```python
from build123d import *

# Parameters (mm, degrees)
SKETCH_1_W               = 120
SKETCH_1_H               = 15
EXTRUDE_1_DEPTH          = 8
FILLET_1_R               = 5
SKETCH_6_R               = 12.5
EXTRUDE_2_DEPTH          = 8
SKETCH_7_R               = 1
CUT_EXTRUDE_4_DEPTH      = 23
SKETCH_8_R               = 2.4
CUT_EXTRUDE_5_DEPTH      = 23
SKETCH_9_W               = 8
SKETCH_9_H               = 15
EXTRUDE_3_DEPTH          = 100
SKETCH_10_W              = 25
SKETCH_10_H              = 6
CUT_EXTRUDE_6_DEPTH      = 5
CUT_EXTRUDE_7_DEPTH      = 7
CUT_EXTRUDE_7_DEPTH_BACK = 15
SKETCH_4_R               = 1
FILLET_2_R               = 10
FILLET_4_R               = 5
CUT_EXTRUDE_8_REACH      = 123.918
SKETCH_12_R              = 1


with BuildPart() as part:
    # 草图1 → 凸台-拉伸1 (new body)
    with BuildSketch(Plane(origin=(0, 0, 0), x_dir=(0, 0, -1), z_dir=(1, 0, 0))):
        with Locations((60, 7.5)):
            Rectangle(SKETCH_1_W, SKETCH_1_H)
    extrude(amount=EXTRUDE_1_DEPTH)

    # 圆角1
    fillet_1_edges = [part.edges().sort_by_distance(p)[0] for p in [
        (4, 15, 0),
        (4, 15, -120),
        (4, 0, -120),
        (4, 0, 0),
    ]]
    fillet(fillet_1_edges, radius=FILLET_1_R)

    # 草图6 → 凸台-拉伸2 (add)
    with BuildSketch(Plane(origin=(8, 0, 0), x_dir=(0, 0, -1), z_dir=(1, 0, 0))):
        with Locations((6.4, 7.5)):
            Circle(SKETCH_6_R)
    extrude(amount=-EXTRUDE_2_DEPTH)

    # 草图7 → 切除-拉伸4 (cut)
    with BuildSketch(Plane.ZY):
        with Locations((-6.4, 12.5)):
            Circle(SKETCH_7_R)
        with Locations((-6.4, 2.5)):
            Circle(SKETCH_7_R)
    extrude(amount=-CUT_EXTRUDE_4_DEPTH, mode=Mode.SUBTRACT)

    # 草图8 → 切除-拉伸5 (cut)
    with BuildSketch(Plane.ZY):
        with Locations((-6.4, 7.5)):
            Circle(SKETCH_8_R)
    extrude(amount=-CUT_EXTRUDE_5_DEPTH, mode=Mode.SUBTRACT)

    # 草图9 → 凸台-拉伸3 (add)
    with BuildSketch(Plane.XY):
        with Locations((4, 7.5)):
            Rectangle(SKETCH_9_W, SKETCH_9_H)
    extrude(amount=EXTRUDE_3_DEPTH)

    # 草图10 → 切除-拉伸6 (cut)
    with BuildSketch(Plane.ZY):
        with Locations((16.022995474, 7.5)):
            Rectangle(SKETCH_10_W, SKETCH_10_H)
    extrude(amount=-CUT_EXTRUDE_6_DEPTH, mode=Mode.SUBTRACT)

    # 草图4 → 切除-拉伸7 (cut, two sides: drawn at the far end of the back side and taken through both)
    with BuildSketch(Plane.XY.offset(-CUT_EXTRUDE_7_DEPTH_BACK)):
        with Locations(Location((2.5, 7.5, 0), (0, 0, 180.000000002))):
            Circle(SKETCH_4_R)
    extrude(amount=CUT_EXTRUDE_7_DEPTH + CUT_EXTRUDE_7_DEPTH_BACK, mode=Mode.SUBTRACT)

    # 圆角2
    fillet_2_edges = [part.edges().sort_by_distance(p)[0] for p in [
        (4, 0, -16.4),
        (4, 15, -16.4),
        (4, 15, 3.6),
        (4, 0, 3.6),
    ]]
    fillet(fillet_2_edges, radius=FILLET_2_R)

    # 圆角4
    fillet_4_edges = [part.edges().sort_by_distance(p)[0] for p in [
        (4, 0, 100),
        (4, 15, 100),
    ]]
    fillet(fillet_4_edges, radius=FILLET_4_R)

    # 草图12 → 切除-拉伸8 (cut, up to next)
    with BuildSketch(Plane.ZY, mode=Mode.PRIVATE) as cut_extrude_8_sk1:
        with Locations((-115, 7.5)):
            Circle(SKETCH_12_R)
    cut_extrude_8_tool1 = extrude(cut_extrude_8_sk1.sketch, amount=-CUT_EXTRUDE_8_REACH, mode=Mode.PRIVATE) & part.part
    # 草图12 → 切除-拉伸8 (cut, up to next)
    with BuildSketch(Plane.ZY, mode=Mode.PRIVATE) as cut_extrude_8_sk2:
        with Locations((-105, 7.5)):
            Circle(SKETCH_12_R)
    cut_extrude_8_tool2 = extrude(cut_extrude_8_sk2.sketch, amount=-CUT_EXTRUDE_8_REACH, mode=Mode.PRIVATE) & part.part
    # 草图12 → 切除-拉伸8 (cut, up to next)
    with BuildSketch(Plane.ZY, mode=Mode.PRIVATE) as cut_extrude_8_sk3:
        with Locations((-82, 7.5)):
            Circle(SKETCH_12_R)
    cut_extrude_8_tool3 = extrude(cut_extrude_8_sk3.sketch, amount=-CUT_EXTRUDE_8_REACH, mode=Mode.PRIVATE) & part.part
    # 草图12 → 切除-拉伸8 (cut, up to next)
    with BuildSketch(Plane.ZY, mode=Mode.PRIVATE) as cut_extrude_8_sk4:
        with Locations((-72, 7.5)):
            Circle(SKETCH_12_R)
    cut_extrude_8_tool4 = extrude(cut_extrude_8_sk4.sketch, amount=-CUT_EXTRUDE_8_REACH, mode=Mode.PRIVATE) & part.part
    # 草图12 → 切除-拉伸8 (cut, up to next)
    with BuildSketch(Plane.ZY, mode=Mode.PRIVATE) as cut_extrude_8_sk5:
        with Locations((95, 7.5)):
            Circle(SKETCH_12_R)
    cut_extrude_8_tool5 = extrude(cut_extrude_8_sk5.sketch, amount=-CUT_EXTRUDE_8_REACH, mode=Mode.PRIVATE) & part.part
    # 草图12 → 切除-拉伸8 (cut, up to next)
    with BuildSketch(Plane.ZY, mode=Mode.PRIVATE) as cut_extrude_8_sk6:
        with Locations((85, 7.5)):
            Circle(SKETCH_12_R)
    cut_extrude_8_tool6 = extrude(cut_extrude_8_sk6.sketch, amount=-CUT_EXTRUDE_8_REACH, mode=Mode.PRIVATE) & part.part
    add(cut_extrude_8_tool1.solids().sort_by_distance((0, 7.5, -115))[0], mode=Mode.SUBTRACT)
    add(cut_extrude_8_tool2.solids().sort_by_distance((0, 7.5, -105))[0], mode=Mode.SUBTRACT)
    add(cut_extrude_8_tool3.solids().sort_by_distance((0, 7.5, -82))[0], mode=Mode.SUBTRACT)
    add(cut_extrude_8_tool4.solids().sort_by_distance((0, 7.5, -72))[0], mode=Mode.SUBTRACT)
    add(cut_extrude_8_tool5.solids().sort_by_distance((0, 7.5, 95))[0], mode=Mode.SUBTRACT)
    add(cut_extrude_8_tool6.solids().sort_by_distance((0, 7.5, 85))[0], mode=Mode.SUBTRACT)


solid = part.part
```
Design review of the part built by this model. Coordinates are the model's own, in mm. A direction names the side the tool comes from. Give positions to 0.01 mm unless a question says otherwise; leave off trailing zeros. Write each loop counter-clockwise with the first axis right and the second up, starting at its lowest first coordinate (ties: lowest second). Pieces come first, ordered by that corner, then holes. Notation, with made-up numbers: (87.25, 64.25) -> (116.25, 64.25) arc R6 cw to (116.25, 72.25) -> close; hole circle Ø1 at (43, -20). An arc over 180 degrees is marked (long way). Answer in a Markdown table with one row per item.
(1) Consider section B-B (z = 72). State the section outline as (x, y) points.
Results:
| item | result |
|---|---|
| outline | (0, 0) -> (8, 0) -> (8, 15) -> (0, 15) -> close |
(2) To check wall thickness, follow probe 1 along Y at (x, z) = (6, -6.4); probe 2 along X at (y, z) = (7.5, -13.5); probe 3 along Y at (x, z) = (3.25, -61). State the ranges of each line that lie inside material, in increasing order.
Results:
| item | result |
|---|---|
| probe 1 | -5 to 1.5, 3.5 to 5.1, 9.9 to 11.5, 13.5 to 20 |
| probe 2 | 0 to 1.5, 3.5 to 8 |
| probe 3 | 0 to 15 |
(3) For faces 4 (the flat face through (5, 8, 16)), 5 (the flat face through (4, 0, -67)), 6 (the flat face through (4, 0, 51)), 7 (the cylindrical face through (4.06, 15.59, 4.36)), 8 (the flat face through (4, 15, -67)), list the 3-axis set-ups (+Z, -Z, +X, -X, +Y, -Y) from which the entire face can be reached by the end or side of a thin tool; tool diameter is ignored.
Results:
| item | result |
|---|---|
| face 4 | -X |
| face 5 | -Z, +X, -X, -Y |
| face 6 | +Z, +X, -X, -Y |
| face 7 | +Z, +X, -X, +Y |
| face 8 | -Z, +X, -X, +Y |
(4) Consider section A-A (z = 14). State the section outline as (x, y) points, then the cut area to 3 significant figures.
Results:
| item | result |
|---|---|
| outline | (0, 0) -> (8, 0) -> (8, 15) -> (0, 15) -> (0, 10.5) -> (5, 10.5) -> (5, 4.5) -> (0, 4.5) -> close |
| area | 90.0 mm2 |
(5) Clearance check with flat-ended pins moving along their axes: pin 1 (2.5 mm diameter, centred on y = 7.5, z = 85, fed in from -X); pin 2 (1.2 mm diameter, centred on y = 12.5, z = -6.4, fed in from +X); pin 3 (3 mm diameter, centred on y = 7.5, z = 20.5, fed in from -X); pin 4 (3 mm diameter, centred on x = 6.5, y = 2.5, fed in from +Z). State where each tip first meets the part, or that it passes through.
Results:
| item | result |
|---|---|
| pin 1 | x = 0 |
| pin 2 | through |
| pin 3 | x = 5 |
| pin 4 | z = 99.9 |
(6) Mouldability with a two-part tool opening along Z and no side actions: class faces 1 (the flat face through (0, 10, -8)), 2 (the cylindrical face through (4.056, 15.556, -17.254)), 3 (the flat face through (2, 7, 28.523)) as +Z half, -Z half, draft (parallel to the pull), parting line (faces both ways), or undercut.
Results:
| item | result |
|---|---|
| face 1 | draft |
| face 2 | -Z half |
| face 3 | undercut |
